The drawing under review shows one solid part. Ordinate dimensions are in mm from its lowest x, y, z. Give positions to 0.01 mm unless a question says otherwise; leave off trailing zeros. Order: outer loops, then holes, each group sorted by start corner. A loop starts at its lowest first (then second) coordinate and runs counter-clockwise, first axis right, second up. Notation, with made-up numbers: (68.5, 45.25) - (82.5, 45.25) arc R19 cw to (82.5, 74.25) - close; hole circle Ø7 at (2.5, -21.5). An arc over 180 degrees is marked (long way). Write item = value, one per line. Start each with the question number.
1. Mouldability with a two-part tool opening along X and no side actions: class the marked faces 1, 2, 3 and 4 as pulls with the +X half, pulls with the -X half, needs draft (parallel to the pull), parting line crosses it, or undercut.
2. We need section B-B, the plane z = 11.5. Give the boundary of the cut face in (x, y).
3. We need section A-A, the plane x = 150. Give the boundary of the cut face in (y, z), and give its area (3 significant figures).
4. Wall thickness on probe 1 along Y at (x, z) = (150, 12); probe 2 along Y at (x, z) = (140.5, 10.5); probe 3 along X at (y, z) = (60, 39): over which ranges is each line inside the solid? List them lowest first.
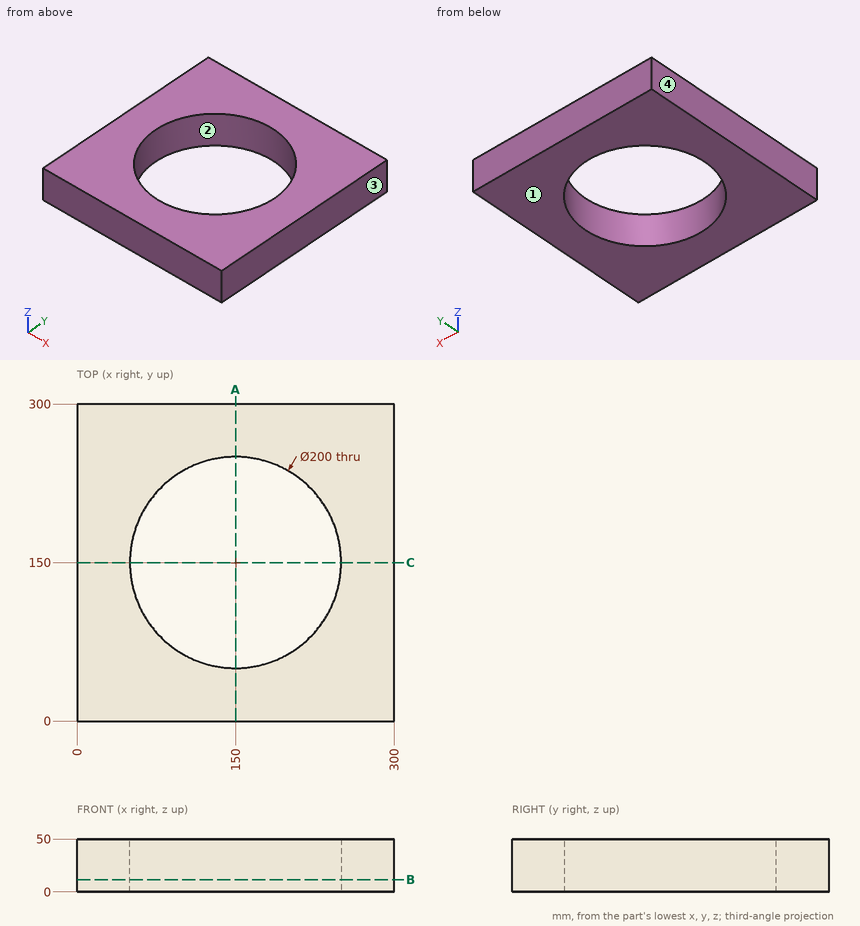
Model answer:
q1.face_1 = needs draft
q1.face_2 = undercut
q1.face_3 = pulls with the +X half
q1.face_4 = pulls with the -X half
q2.outline = (0, 0) - (300, 0) - (300, 300) - (0, 300) - close; hole circle Ø200 at (150, 150)
q3.outline = (0, 0) - (50, 0) - (50, 50) - (0, 50) - close; (250, 0) - (300, 0) - (300, 50) - (250, 50) - close
q3.area = 5,000 mm2
q4.probe_1 = 0 to 50, 250 to 300
q4.probe_2 = 0 to 50.45, 249.55 to 300
q4.probe_3 = 0 to 106.41, 193.59 to 300
